from build123d import *

# Parameters (mm, degrees)
BOSS_EXTRUDE1_DEPTH = 25
SKETCH3_R           = 5
CUT_EXTRUDE1_DEPTH  = 30
SKETCH8_W           = 15
SKETCH8_H           = 3
CUT_EXTRUDE10_DEPTH = 30
FILLET1_R           = 1
FILLET2_R           = 1


with BuildPart() as part:
    # Sketch2 → Boss-Extrude1 (new body)
    with BuildSketch(Plane(origin=(0, 0, 0), x_dir=(0, 0, -1), z_dir=(1, 0, 0))):
        Polygon((25, 40.957602214), (53.678821818, 40.957602214), (25, 0), (0, 0), (0, 40.957602214), align=None)
    extrude(amount=BOSS_EXTRUDE1_DEPTH)

    # Sketch3 → Cut-Extrude1 (cut)
    with BuildSketch(Plane.XZ):
        with Locations(Location((12.5, -12.5, 0), (0, 0, 270))):
            Circle(SKETCH3_R)
    extrude(amount=-CUT_EXTRUDE1_DEPTH, mode=Mode.SUBTRACT)

    # Sketch8 → Cut-Extrude10 (cut)
    with BuildSketch(Plane.XY.offset(-15)):
        with Locations((12.5, 5.957602214)):
            Rectangle(SKETCH8_W, SKETCH8_H)
    extrude(amount=-CUT_EXTRUDE10_DEPTH, mode=Mode.SUBTRACT)

    # Fillet1
    fillet1_edges = [part.edges().sort_by_distance(p)[0] for p in [
        (25, 0, -12.5),
        (25, 20.478801107, -39.339410909),
        (5, 5.957602214, -29.17155798),
        (20, 5.957602214, -29.17155798),
        (12.5, 4.457602214, -28.121246673),
        (12.5, 7.457602214, -30.221869288),
        (25, 40.957602214, -26.839410909),
        (0, 40.957602214, -26.839410909),
        (0, 20.478801107, -39.339410909),
        (0, 0, -12.5),
        (0, 20.478801107, 0),
        (25, 20.478801107, 0),
        (12.5, 40.957602214, -53.678821818),
        (12.5, 0, -25),
        (12.5, 0, 0),
        (12.5, 40.957602214, 0),
    ]]
    fillet(fillet1_edges, radius=FILLET1_R)

    # Fillet2
    fillet2_edges = [part.edges().sort_by_distance(p)[0] for p in [
        (12.5, 0, -7.5),
    ]]
    fillet(fillet2_edges, radius=FILLET2_R)


solid = part.part
Geometry: final body of the model. Coordinates: model frame, mm. A direction names the side the tool comes from. Give positions to 0.01 mm unless a question says otherwise; leave off trailing zeros. Write each loop counter-clockwise with the first axis right and the second up, starting at its lowest first coordinate (ties: lowest second). Pieces come first, ordered by that corner, then holes.
(1) Access query for faces 1 (the flat face through (13, 30, -12)), 2 (the flat face through (12, 20, 0)), 3 (the flat face through (7, 6, -15)). Directions: +Z, -Z, +X, -X, +Y, -Y. A direction counts if a zero-diameter tool reaches every point of the face in a straight line with its end or side. Return the directions, or none.
(2) Cut plane B-B, the plane z = -12.5. Return loops of the section in (x, y), then the cut area to 3 significant figures.
(3) Cut plane A-A, the plane x = 12.5. Return loops of the section in (y, z), then the cut area to 3 significant figures.
(4) Ray query, line 1 (X direction, y = 14.5, z = -12.5); line 2 (Y direction, x = 8.5, z = -14); line 3 (Z direction, x = 8.5, y = 9). Return the intervals inside material, ascending.
(5) First-contact query: P1, Ø6, axis at x = 14, z = -42, coming from the -Y side; P2, Ø0.9, axis at x = 6, y = 6.5, coming from the -Z side; P3, Ø3.5, axis at x = 18.5, y = 6.5, coming from the -Z side. Flat tips, straight axial feed; report the tip coordinate or a pass-through.
(6) Mould query, pull axis X, two halves, no side actions, for faces 4 (the flat face through (20, 6, -22)), 5 (the flat face through (12, 40.958, -27)), 6 (the cylindrical face through (4.7, 5.5, -28.5)), 7 (the flat face through (0, 25, -21)). Classes: released by +X, released by -X, zero draft, split by the parting line, or undercut.
Values follow:
1. face 1: -Y
1. face 2: +Z, +X, -X, +Y, -Y
1. face 3: -Z
2. outline: (0, 1) arc R1 ccw to (1, 0) - (6.5, 0) arc R1 ccw to (7.5, 1) - (7.5, 30) - (17.5, 30) - (17.5, 1) arc R1 ccw to (18.5, 0) - (24, 0) arc R1 ccw to (25, 1) - (25, 39.96) arc R1 ccw to (24, 40.96) - (1, 40.96) arc R1 ccw to (0, 39.96) - close
2. area: 723 mm2
3. outline: (0, -24.48) arc R1 ccw to (0.43, -25.3) - (2.88, -27.02) arc R1 ccw to (4.46, -26.2) - (4.46, -17.5) - (1, -17.5) arc R1 ccw to (0, -18.5) - close; (0, -6.5) arc R1 ccw to (1, -7.5) - (30, -7.5) - (30, -17.5) - (7.46, -17.5) - (7.46, -29.7) arc R1 ccw to (7.88, -30.52) - (39.38, -52.58) arc R1 ccw to (40.96, -51.76) - (40.96, -1) arc R1 ccw to (39.96, 0) - (1, 0) arc R1 ccw to (0, -1) - close
3. area: 1,270 mm2
4. line 1: x = 0 to 7.5, 17.5 to 25
4. line 2: y = 30 to 40.96
4. line 3: z = -31.3 to -15.5, -9.5 to 0
5. P1: stops at y = 19.99
5. P2: stops at z = -15
5. P3: stops at z = -30.78
6. face 4: undercut
6. face 5: zero draft
6. face 6: undercut
6. face 7: released by -X
